```python
from build123d import *

# Parameters (mm, degrees)
SKETCH1_R           = 2
SKETCH1_R_2         = 5.25
BOSS_EXTRUDE1_DEPTH = 4


with BuildPart() as part:
    # Sketch1 → Boss-Extrude1 (new body)
    with BuildSketch(Plane(origin=(0, 0, 0), x_dir=(1, 0, 0), z_dir=(0, 1, 0))):
        with BuildLine():
            Line((316.226041149, 107.292047617), (316.226041149, -261.707952383))
            ThreePointArc((316.226041149, -261.707952383), (317.104720805, -263.829272726), (319.226041149, -264.707952383))
            Line((319.226041149, -264.707952383), (653.226041149, -264.707952383))
            ThreePointArc((653.226041149, -264.707952383), (655.347361492, -263.829272726), (656.226041149, -261.707952383))
            Line((656.226041149, -261.707952383), (656.226041149, 107.292047617))
            ThreePointArc((656.226041149, 107.292047617), (655.347361492, 109.413367961), (653.226041149, 110.292047617))
            Line((653.226041149, 110.292047617), (319.226041149, 110.292047617))
            ThreePointArc((319.226041149, 110.292047617), (317.104720805, 109.413367961), (316.226041149, 107.292047617))
        make_face()
        with Locations((450.618955235, -162.614244131)):
            Circle(SKETCH1_R, mode=Mode.SUBTRACT)
        with Locations((440.618955235, -162.614244131)):
            Circle(SKETCH1_R, mode=Mode.SUBTRACT)
        with Locations((517.330184073, -178.73741306)):
            Circle(SKETCH1_R, mode=Mode.SUBTRACT)
        with Locations((644.226041149, -77.207952383)):
            Circle(SKETCH1_R_2, mode=Mode.SUBTRACT)
        with Locations((328.226041149, -77.207952383)):
            Circle(SKETCH1_R_2, mode=Mode.SUBTRACT)
        with Locations((644.226041149, 94.292047617)):
            Circle(SKETCH1_R_2, mode=Mode.SUBTRACT)
        with Locations((328.226041149, 94.292047617)):
            Circle(SKETCH1_R_2, mode=Mode.SUBTRACT)
        with Locations((328.226041149, -248.707952383)):
            Circle(SKETCH1_R_2, mode=Mode.SUBTRACT)
        with Locations((644.226041149, -248.707952383)):
            Circle(SKETCH1_R_2, mode=Mode.SUBTRACT)
        with Locations((527.330184073, -178.73741306)):
            Circle(SKETCH1_R, mode=Mode.SUBTRACT)
    extrude(amount=BOSS_EXTRUDE1_DEPTH)


solid = part.part
```
Design review of the part built by this model. Coordinates are the model's own, in mm. Coordinates: 2 decimals unless noted, no trailing zeros.
Q1. For pin 1 (13.5 mm diameter, centred on x = 328.23, z = 248.71, fed in from -Y); pin 2 (6.5 mm diameter, centred on x = 644.23, z = -94.29, fed in from +Y), all flat-tipped, find the tip position at first contact; note any pin that passes through.
Reported:
pin 1: stops at y = 0
pin 2: passes through
Q2. To check wall thickness, follow line 1 (X direction, y = 1.5, z = 161); line 2 (Z direction, x = 529, y = 0.6). State the ranges of each line that lie inside material, in increasing order.
Reported:
line 1: x = 316.23 to 439.44, 441.8 to 449.44, 451.8 to 656.23
line 2: z = -110.29 to 177.64, 179.84 to 264.71
Q3. The part is to be moulded in two halves that separate along Z. For faces 1 (the face through (649.076, 1.972, 250.719)), 2 (the face through (484, 4, 75)), say which applies: +Z half, -Z half, draft (parallel to the pull), parting line (faces both ways), or undercut.
Reported:
face 1: undercut
face 2: draft
